The listing builds one solid part. Answer for the finished solid, in the listing's coordinates (mm). Face numbers are marked on the shaded views. Give positions to 0.01 mm unless a question says otherwise; leave off trailing zeros. Order: outer loops, then holes, each group sorted by start corner. A loop starts at its lowest first (then second) coordinate and runs counter-clockwise, first axis right, second up. Notation, with made-up numbers: (22.25, 42.5) -> (52.25, 42.5) arc R36 cw to (52.25, 79.5) -> close; hole circle Ø6 at (12.5, -19). An arc over 180 degrees is marked (long way). Write item = value, one per line. Start each with the question number.
```python
from build123d import *

# Parameters (mm, degrees)
SZKIC1_W                    = 387
SZKIC1_H                    = 1.75
DODANIE_WYCI_GNI_CIE1_DEPTH = 290
DODANIE_WYCI_GNI_CIE2_DEPTH = 20


with BuildPart() as part:
    # Szkic1 → Dodanie-wyciągnięcie1 (new body)
    with BuildSketch(Plane.XY):
        with Locations((0, -0.875)):
            Rectangle(SZKIC1_W, SZKIC1_H)
    extrude(amount=DODANIE_WYCI_GNI_CIE1_DEPTH)

    # Szkic2 → Dodanie-wyciągnięcie2 (add)
    with BuildSketch(Plane.XZ.offset(1.75)):
        Polygon((-193.5, 290), (-193.5, 0), (193.5, 0), (193.5, 290), (191.75, 290), (191.75, 1.75), (-191.75, 1.75), (-191.75, 290), align=None)
    extrude(amount=DODANIE_WYCI_GNI_CIE2_DEPTH)


solid = part.part
```
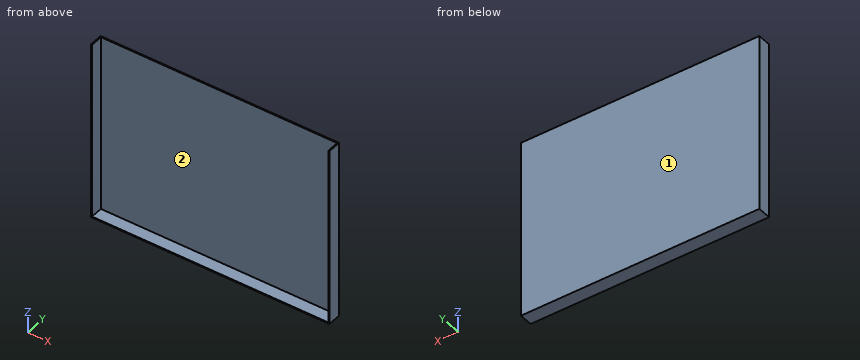
Item 1: Consider L1, parallel to X at y = -11, z = 20; L2, parallel to Y at x = 119.5, z = 272.5; L3, parallel to Z at x = -164, y = -13.25. Determine where each line is inside the solid, lowest interval first. Write a range as from..to.
Item 2: A cutting plane is placed at C-C, the plane z = 252.5. Write down the section's boundary in (x, y), plus the area to 3 significant figures.
Item 3: A cutting plane is placed at A-A, the plane y = -18. Write down the section's boundary in (x, z), plus the area to 3 significant figures.
Item 4: Flat-ended cylindrical pins translate along their axes: pin 1 (5 mm diameter, centred on x = 101.5, y = -7.5, fed in from -Z); pin 2 (2 mm diameter, centred on x = -48.5, y = -15, fed in from +Z); pin 3 (12 mm diameter, centred on x = -96.5, z = 215, fed in from -Y). Find the tip coordinate at first contact, or state that the pin passes through.
Item 5: The mould has two halves that part along Y. Classify the marked faces 1 and 2: +Y half, -Y half, draft (parallel to the pull), parting line (faces both ways), or undercut.
Item 6: A cutting plane is placed at B-B, the plane x = 106. Write down the section's boundary in (y, z), plus the area to 4 significant figures.
Check values:
q1.L1 = -193.5..-191.75, 191.75..193.5
q1.L2 = -1.75..0
q1.L3 = 0..1.75
q2.outline = (-193.5, -21.75) -> (-191.75, -21.75) -> (-191.75, -1.75) -> (191.75, -1.75) -> (191.75, -21.75) -> (193.5, -21.75) -> (193.5, 0) -> (-193.5, 0) -> close
q2.area = 747 mm^2
q3.outline = (-193.5, 0) -> (193.5, 0) -> (193.5, 290) -> (191.75, 290) -> (191.75, 1.75) -> (-191.75, 1.75) -> (-191.75, 290) -> (-193.5, 290) -> close
q3.area = 1,690 mm^2
q4.pin_1 = 0
q4.pin_2 = 1.75
q4.pin_3 = -1.75
q5.face_1 = +Y half
q5.face_2 = -Y half
q6.outline = (-21.75, 0) -> (0, 0) -> (0, 290) -> (-1.75, 290) -> (-1.75, 1.75) -> (-21.75, 1.75) -> close
q6.area = 542.5 mm^2
